from build123d import *

# Parameters (mm, degrees)
BOSS_EXTRUDE1_DEPTH     = 40
SKETCH2_R               = 12.5
CUT_EXTRUDE1_DEPTH      = 4.4775
FILLET1_R               = 10
CUT_EXTRUDE2_DEPTH      = 131.2
CUT_EXTRUDE2_DEPTH_BACK = 14.2
SKETCH4_R               = 2.5
SKETCH6_W               = 68
SKETCH6_H               = 90
BOSS_EXTRUDE4_DEPTH     = 10
FILLET2_R               = 10
FILLET3_R               = 5
FILLET4_R               = 4
CUT_EXTRUDE3_START      = -2.2025
SKETCH7_R               = 3.9
CUT_EXTRUDE3_DEPTH      = 0.85
SKETCH8_R               = 3.25
CUT_EXTRUDE4_DEPTH      = 10
SKETCH9_R               = 4.025
CUT_EXTRUDE5_DEPTH      = 12
SKETCH10_W              = 20.05
SKETCH10_H              = 20.05
CUT_EXTRUDE6_DEPTH      = 4
CUT_EXTRUDE7_DEPTH      = 6
CUT_EXTRUDE9_DEPTH      = 2.5
CUT_EXTRUDE10_REACH     = 138.104
CUT_EXTRUDE10_START     = 2.5
SKETCH15_R              = 1.5


with BuildPart() as part:
    # Sketch1 → Boss-Extrude1 (new body)
    with BuildSketch(Plane.XY):
        Polygon((10, 0), (10, 43), (104, 43), (104, 0), (114, 0), (114, 53), (0, 53), (0, 0), align=None)
    extrude(amount=-BOSS_EXTRUDE1_DEPTH)

    # Sketch2 → Cut-Extrude1 (cut)
    with BuildSketch(Plane(origin=(10, 0, 0), x_dir=(0, 0, -1), z_dir=(1, 0, 0))):
        with Locations((20, 19.635146369)):
            Circle(SKETCH2_R)
    extrude(amount=-CUT_EXTRUDE1_DEPTH, mode=Mode.SUBTRACT)

    # Fillet1
    fillet1_edges = [part.edges().sort_by_distance(p)[0] for p in [
        (5, 0, 0),
        (109, 0, -40),
        (5, 0, -40),
        (109, 0, 0),
    ]]
    fillet(fillet1_edges, radius=FILLET1_R)

    # Sketch4 → Cut-Extrude2 (cut, two sides: drawn at the far end of the back side and taken through both)
    with BuildSketch(Plane(origin=(7.725, 0, 0), x_dir=(0, 0, -1), z_dir=(1, 0, 0)).offset(-CUT_EXTRUDE2_DEPTH_BACK)):
        with Locations(Location((20, 19.635146369, 0), (0, 0, 180))):
            Circle(SKETCH4_R)
    extrude(amount=CUT_EXTRUDE2_DEPTH + CUT_EXTRUDE2_DEPTH_BACK, mode=Mode.SUBTRACT)

    # Sketch6 → Boss-Extrude4 (add)
    with BuildSketch(Plane(origin=(0, 53, 0), x_dir=(1, 0, 0), z_dir=(0, 1, 0))):
        with Locations((57, 20)):
            Rectangle(SKETCH6_W, SKETCH6_H)
    extrude(amount=-BOSS_EXTRUDE4_DEPTH)

    # Fillet2
    fillet2_edges = [part.edges().sort_by_distance(p)[0] for p in [
        (23, 48, 0),
        (91, 48, 0),
        (91, 48, -40),
        (23, 48, -40),
    ]]
    fillet(fillet2_edges, radius=FILLET2_R)

    # Fillet3
    fillet3_edges = [part.edges().sort_by_distance(p)[0] for p in [
        (23, 48, 25),
        (91, 48, -65),
        (91, 48, 25),
        (23, 48, -65),
    ]]
    fillet(fillet3_edges, radius=FILLET3_R)

    # Fillet4
    fillet4_edges = [part.edges().sort_by_distance(p)[0] for p in [
        (0, 53, -20),
        (114, 53, -20),
    ]]
    fillet(fillet4_edges, radius=FILLET4_R)

    # Sketch7 → Cut-Extrude3 (cut)
    with BuildSketch(Plane(origin=(7.725, 0, 0), x_dir=(0, 0, -1), z_dir=(1, 0, 0)).offset(CUT_EXTRUDE3_START)):
        with Locations((20, 19.635146369)):
            Circle(SKETCH7_R)
    extrude(amount=-CUT_EXTRUDE3_DEPTH, mode=Mode.SUBTRACT)

    # Sketch8 → Cut-Extrude4 (cut)
    with BuildSketch(Plane(origin=(0, 53, 0), x_dir=(1, 0, 0), z_dir=(0, 1, 0))):
        with Locations(Location((57, 20, 0), (0, 0, 270))):
            Circle(SKETCH8_R)
    extrude(amount=-CUT_EXTRUDE4_DEPTH, mode=Mode.SUBTRACT)

    # Sketch9 → Cut-Extrude5 (cut)
    with BuildSketch(Plane(origin=(114, 0, 0), x_dir=(0, 0, -1), z_dir=(1, 0, 0))):
        with Locations(Location((20, 19.635146369, 0), (0, 0, 90))):
            Circle(SKETCH9_R)
    extrude(amount=-CUT_EXTRUDE5_DEPTH, mode=Mode.SUBTRACT)

    # Sketch10 → Cut-Extrude6 (cut)
    with BuildSketch(Plane(origin=(114, 0, 0), x_dir=(0, 0, -1), z_dir=(1, 0, 0))):
        with Locations((20, 19.635146369)):
            Rectangle(SKETCH10_W, SKETCH10_H)
    extrude(amount=-CUT_EXTRUDE6_DEPTH, mode=Mode.SUBTRACT)

    # Sketch14 → Cut-Extrude7 (cut)
    with BuildSketch(Plane(origin=(0, 53, 0), x_dir=(1, 0, 0), z_dir=(0, 1, 0))):
        Polygon((56.872881106, 25.694991584), (61.872881106, 22.808240238), (61.872881106, 17.034737546), (56.872881106, 14.1479862), (51.872881106, 17.034737546), (51.872881106, 22.808240238), align=None)
    extrude(amount=-CUT_EXTRUDE7_DEPTH, mode=Mode.SUBTRACT)

    # Sketch18 → Cut-Extrude9 (cut)
    with BuildSketch(Plane.ZY.offset(-104)):
        Polygon((-15.048857438, 28.91356654), (-11.910134999, 28.91356654), (-10.270487153, 26.081726401), (-11.891583597, 23.249886262), (-15.151000849, 23.249886262), (-16.733963505, 26.081726401), align=None)
        Polygon((-23.266036495, 26.081726401), (-24.951142562, 28.91356654), (-28.089865001, 28.91356654), (-29.729512847, 26.081726401), (-28.108416403, 23.249886262), (-24.848999151, 23.249886262), align=None)
        Polygon((-16.733963505, 13.188566337), (-15.048857438, 10.356726198), (-11.910134999, 10.356726198), (-10.270487153, 13.188566337), (-11.891583597, 16.020406476), (-15.151000849, 16.020406476), align=None)
        Polygon((-24.848999151, 16.020406476), (-23.266036495, 13.188566337), (-24.951142562, 10.356726198), (-28.089865001, 10.356726198), (-29.729512847, 13.188566337), (-28.108416403, 16.020406476), align=None)
    extrude(amount=-CUT_EXTRUDE9_DEPTH, mode=Mode.SUBTRACT)

    # Sketch15 → Cut-Extrude10 (cut, up to next)
    with BuildSketch(Plane.ZY.offset(-104).offset(CUT_EXTRUDE10_START), mode=Mode.PRIVATE) as cut_extrude10_sk1:
        with Locations(Location((-26.5, 26.135146369, 0), (0, 0, 270))):
            Circle(SKETCH15_R)
    cut_extrude10_tool1 = extrude(cut_extrude10_sk1.sketch, amount=-CUT_EXTRUDE10_REACH, mode=Mode.PRIVATE) & part.part
    # Sketch15 → Cut-Extrude10 (cut, up to next)
    with BuildSketch(Plane.ZY.offset(-104).offset(CUT_EXTRUDE10_START), mode=Mode.PRIVATE) as cut_extrude10_sk2:
        with Locations(Location((-13.5, 26.135146369, 0), (0, 0, 270))):
            Circle(SKETCH15_R)
    cut_extrude10_tool2 = extrude(cut_extrude10_sk2.sketch, amount=-CUT_EXTRUDE10_REACH, mode=Mode.PRIVATE) & part.part
    # Sketch15 → Cut-Extrude10 (cut, up to next)
    with BuildSketch(Plane.ZY.offset(-104).offset(CUT_EXTRUDE10_START), mode=Mode.PRIVATE) as cut_extrude10_sk3:
        with Locations(Location((-13.5, 13.135146369, 0), (0, 0, 270))):
            Circle(SKETCH15_R)
    cut_extrude10_tool3 = extrude(cut_extrude10_sk3.sketch, amount=-CUT_EXTRUDE10_REACH, mode=Mode.PRIVATE) & part.part
    # Sketch15 → Cut-Extrude10 (cut, up to next)
    with BuildSketch(Plane.ZY.offset(-104).offset(CUT_EXTRUDE10_START), mode=Mode.PRIVATE) as cut_extrude10_sk4:
        with Locations(Location((-26.5, 13.135146369, 0), (0, 0, 270))):
            Circle(SKETCH15_R)
    cut_extrude10_tool4 = extrude(cut_extrude10_sk4.sketch, amount=-CUT_EXTRUDE10_REACH, mode=Mode.PRIVATE) & part.part
    add(cut_extrude10_tool1.solids().sort_by_distance((101.5, 26.135146, -26.5))[0], mode=Mode.SUBTRACT)
    add(cut_extrude10_tool2.solids().sort_by_distance((101.5, 26.135146, -13.5))[0], mode=Mode.SUBTRACT)
    add(cut_extrude10_tool3.solids().sort_by_distance((101.5, 13.135146, -13.5))[0], mode=Mode.SUBTRACT)
    add(cut_extrude10_tool4.solids().sort_by_distance((101.5, 13.135146, -26.5))[0], mode=Mode.SUBTRACT)


solid = part.part
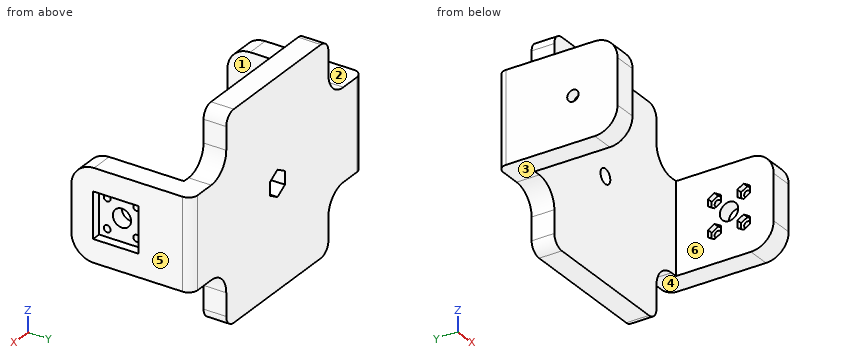
Read the model definition and answer for the solid it produces. Units are mm, in the model's axes. Face numbers are marked on the shaded views. A direction names the side the tool comes from. Give positions to 0.01 mm unless a question says otherwise; leave off trailing zeros. Loops run counter-clockwise (first coordinate to the right, second up) from the corner with the lowest first, then second, coordinate; pieces in that order, holes last. Notation, with made-up numbers: (32.25, 8) -> (70.25, 8) arc R18 cw to (70.25, 38) -> close; hole circle Ø11 at (47.5, 46.5). An arc over 180 degrees is marked (long way). Use a Markdown table: item, result.
Q1. Determine the mould class of the marked faces 4, 5 and 6 for opening direction X: pulls with the +X half, pulls with the -X half, needs draft (parallel to the pull), parting line crosses it, or undercut.
Solved:
| item | result |
|---|---|
| face 4 | needs draft |
| face 5 | pulls with the +X half |
| face 6 | undercut |
Q2. Section C-C, the plane z = -57 is taken. Determine the outline of the cut face in (x, y), then the cut area to 3 significant figures.
Solved:
| item | result |
|---|---|
| outline | (23, 43) -> (91, 43) -> (91, 53) -> (23, 53) -> close |
| area | 680 mm^2 |
Q3. Each of these flat-tipped pins is pushed along its axis until it touches: pin 1 (1.2 mm diameter, centred on x = 112.5, z = -22.5, fed in from +Y); pin 2 (6.5 mm diameter, centred on x = 9.5, y = 26, fed in from -Z); pin 3 (8 mm diameter, centred on y = 49.5, z = 13.5, fed in from +X). Where does it stop, or does it pass through?
Solved:
| item | result |
|---|---|
| pin 1 | stops at y = 52.52 |
| pin 2 | stops at z = -40 |
| pin 3 | stops at x = 91.01 |
Q4. A tool of negligible diameter and unlimited length cuts with its end or side. For the marked faces 1, 2 and 3, from which of +Z, -Z, +X, -X, +Y, -Y can it reach the whole face along a straight path? Write none if from no direction.
Solved:
| item | result |
|---|---|
| face 1 | +Z, -Z, -Y |
| face 2 | +Z, -X, +Y, -Y |
| face 3 | -Z, -X, +Y, -Y |
Q5. Section B-B, the plane z = -20 is taken. Count the separate pieces of the cut face and the enclosed holes in it, then the cut area to 3 significant figures.
Solved:
| item | result |
|---|---|
| separate pieces | 4 |
| enclosed holes | 0 |
| area | 1,640 mm^2 |
Q6. Section A-A, the plane y = 35.5 is taken. Determine the outline of the cut face in (x, z).
Solved:
| item | result |
|---|---|
| outline | (0, -40) -> (10, -40) -> (10, 0) -> (0, 0) -> close; (104, -40) -> (114, -40) -> (114, 0) -> (104, 0) -> close |
Q7. Section D-D, the plane x = 65.5 is taken. Determine the outline of the cut face in (y, z), then the cut area to 3 significant figures.
Solved:
| item | result |
|---|---|
| outline | (43, -65) -> (53, -65) -> (53, 25) -> (43, 25) -> close |
| area | 900 mm^2 |
Q8. Find the intervals of material crossed by line 1 along Y through (x, z) = (8.75, -20); line 2 along X through (y, z) = (26, -19.5); line 3 along Y through (x, z) = (107, -26), in increasing order.
Solved:
| item | result |
|---|---|
| line 1 | y = 0 to 7.14, 32.14 to 53 |
| line 2 | x = 0 to 5.52, 104 to 110 |
| line 3 | y = 0 to 11.72, 14.55 to 24.72, 27.55 to 53 |
